Could you check a few things on this model? Use its own coordinates, in mm. Coordinates: 2 decimals unless noted, no trailing zeros. Loops run counter-clockwise (first coordinate to the right, second up) from the corner with the lowest first, then second, coordinate; pieces in that order, holes last. Notation, with made-up numbers: (73, -13.75) - (78, -13.75) arc R7 cw to (78, -3.75) - close; hole circle Ø5 at (-2, 16.25). An arc over 180 degrees is marked (long way). One line per item, written item: value. Start each with the question number.
(1) If we section it at B-B on z = 0: Write out the boundary of the cut face in (x, y).
(2) I'm going to push flat-ended pins straight in: P1, Ø5, axis at x = 3.5, z = -2, coming from the +Y side; P2, Ø1, axis at x = -2, y = 6, coming from the -Z side; P3, Ø3.5, axis at x = 0, z = 0, coming from the -Y side. Where does each tip first touch, or does it pass through?
(3) If we mould it in two halves opening along Z, with no side actions, what happens to faces 1 (the face through (-3.905, 3.965, 0.867)), 2 (the face through (3, 6.5, -1)), 3 (the face through (0.9, 3.3, 2.86))? For each: pulls with the +Z half, pulls with the -Z half, needs draft (parallel to the pull), parting line crosses it, or undercut.
(4) If I drill on line 1 along X through (y, z) = (4, 0); line 2 along Z through (x, y) = (-0.5, 3.5); line 3 along Z through (x, y) = (-2, 4), over which ranges is the centre line in solid material (lowest first)? Write a range as from..to.
(5) If we section it at C-C on y = 2.5: Write out the boundary of the cut face in (x, z).
(6) If we section it at A-A on x = 0: Write out the boundary of the cut face in (y, z).
(7) If we section it at D-D on y = 0.75: Write out the boundary of the cut face in (x, z).
```python
from build123d import *

# Parameters (mm, degrees)
SKETCH2_R           = 5
BOSS_EXTRUDE1_DEPTH = 1.5
SKETCH3_R           = 4
BOSS_EXTRUDE2_DEPTH = 6.5
SKETCH4_R           = 3
CUT_EXTRUDE1_DEPTH  = 10.604686356


with BuildPart() as part:
    # Sketch2 → Boss-Extrude1 (new body)
    with BuildSketch(Plane(origin=(0, 0, 0), x_dir=(1, 0, 0), z_dir=(0, 1, 0))):
        with Locations(Location((0, 0, 0), (0, 0, 270))):
            Circle(SKETCH2_R)
    extrude(amount=BOSS_EXTRUDE1_DEPTH)

    # Sketch3 → Boss-Extrude2 (add)
    with BuildSketch(Plane.XZ):
        with Locations(Location((0, 0, 0), (0, 0, 270))):
            Circle(SKETCH3_R)
    extrude(amount=-BOSS_EXTRUDE2_DEPTH)

    # Sketch4 → Cut-Extrude1 (cut, through all)
    with BuildSketch(Plane(origin=(0, 6.5, 0), x_dir=(1, 0, 0), z_dir=(0, 1, 0))):
        with Locations(Location((0, 0, 0), (0, 0, 270))):
            Circle(SKETCH4_R)
    extrude(amount=-CUT_EXTRUDE1_DEPTH, mode=Mode.SUBTRACT)


solid = part.part
```
Values:
1. outline: (-5, 0) - (-3, 0) - (-3, 6.5) - (-4, 6.5) - (-4, 1.5) - (-5, 1.5) - close; (3, 0) - (5, 0) - (5, 1.5) - (4, 1.5) - (4, 6.5) - (3, 6.5) - close
2. P1: stops at y = 6.5
2. P2: stops at z = -3.71
2. P3: passes through
3. face 1: parting line crosses it
3. face 2: needs draft
3. face 3: undercut
4. line 1: x = -4..-3, 3..4
4. line 2: z = -3.97..-2.96, 2.96..3.97
4. line 3: z = -3.46..-2.24, 2.24..3.46
5. outline: circle Ø8 at (0, 0); hole circle Ø6 at (0, 0)
6. outline: (0, -5) - (1.5, -5) - (1.5, -4) - (6.5, -4) - (6.5, -3) - (0, -3) - close; (0, 3) - (6.5, 3) - (6.5, 4) - (1.5, 4) - (1.5, 5) - (0, 5) - close
7. outline: circle Ø10 at (0, 0); hole circle Ø6 at (0, 0)
